Source: CAD feature listing. Evaluate the final solid. Frame: model axes, mm. Face numbers are marked on the shaded views. Give positions to 0.01 mm unless a question says otherwise; leave off trailing zeros. Loops run counter-clockwise (first coordinate to the right, second up) from the corner with the lowest first, then second, coordinate; pieces in that order, holes last.
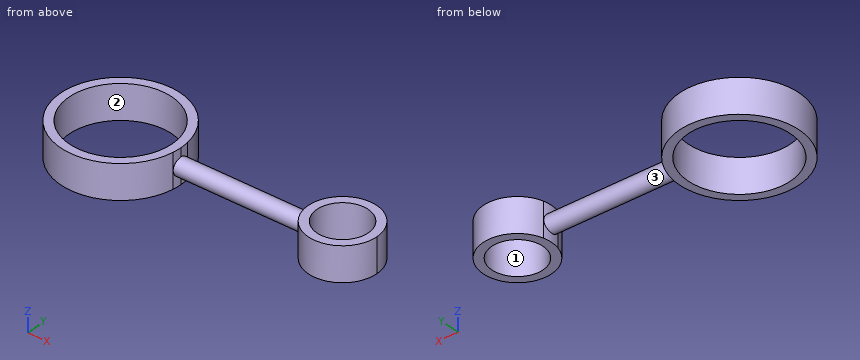
from build123d import *

# Parameters (mm, degrees)
F0_R     = 12.7
F1_DEPTH = 95.25
F2_R     = 76.2
F3_DEPTH = 25.4
F4_R     = 38.1
F5_DEPTH = 25.4


with BuildPart() as f1:
    # F0 (on Right) → F1 (new body, symmetric)
    with BuildSketch(Plane.YZ):
        Circle(F0_R)
    extrude(amount=F1_DEPTH, both=True)

    # F2 (on Top) → F3 (join, symmetric)
    with BuildSketch(Plane.XY):
        with BuildLine():
            ThreePointArc((-94.338181, 0), (-94.566429, 6.366345), (-95.25, 12.7))
            Line((-95.25, 12.7), (-95.25, -12.7))
            ThreePointArc((-95.25, -12.7), (-94.566429, -6.366345), (-94.338181, 0))
        make_face()
        with BuildLine():
            Line((-95.25, -12.7), (-95.25, 12.7))
            ThreePointArc((-95.25, 12.7), (-272.138181, 0), (-95.25, -12.7))
        make_face()
        with Locations((-183.238181, 0)):
            Circle(F2_R, mode=Mode.SUBTRACT)
    extrude(amount=F3_DEPTH, both=True)

    # F4 (on Top) → F5 (join, symmetric)
    with BuildSketch(Plane.XY):
        with BuildLine():
            Line((95.25, -12.7), (95.25, 12.7))
            ThreePointArc((95.25, 12.7), (93.636888, 0), (95.25, -12.7))
        make_face()
        with BuildLine():
            ThreePointArc((195.236888, 0), (150.837907, 50.395109), (95.25, 12.7))
            Line((95.25, 12.7), (95.25, -12.7))
            ThreePointArc((95.25, -12.7), (150.837907, -50.395109), (195.236888, 0))
        make_face()
        with Locations((144.436888, 0)):
            Circle(F4_R, mode=Mode.SUBTRACT)
    extrude(amount=F5_DEPTH, both=True)


solid = f1.part
1) Cut plane A-A (y = 63). Return loops of the section in (x, z), and give its area (3 significant figures).
Checks:
outline: (-245.96, -25.4) - (-226.1, -25.4) - (-226.1, 25.4) - (-245.96, 25.4) - close; (-140.37, -25.4) - (-120.51, -25.4) - (-120.51, 25.4) - (-140.37, 25.4) - close
area: 2,020 mm2
2) Cut plane D-D (z = 6.5). Return loops of the section in (x, y).
Checks:
outline: (-95.25, -12.7) arc R88.9 ccw to (-95.01, -10.91) - (94.82, -10.91) arc R50.8 ccw to (95.25, -12.7) arc R50.8 ccw to (195.24, 0) arc R50.8 ccw to (95.25, 12.7) arc R50.8 ccw to (94.82, 10.91) - (-95.01, 10.91) arc R88.9 ccw to (-95.25, 12.7) arc R88.9 ccw (long way) to start; hole circle Ø152.4 at (-183.24, 0); hole circle Ø76.2 at (144.44, 0)
3) Cut plane B-B (x = -179). Return loops of the section in (y, z), and give its area (3 significant figures).
Checks:
outline: (-88.8, -25.4) - (-76.08, -25.4) - (-76.08, 25.4) - (-88.8, 25.4) - close; (76.08, -25.4) - (88.8, -25.4) - (88.8, 25.4) - (76.08, 25.4) - close
area: 1,290 mm2
4) Contact query for flat-ended pins moving along their axis: P1, Ø12, axis at x = -185, z = -8.5, coming from the +Y side; P2, Ø4, axis at y = -69.5, z = 10, coming from the +X side; P3, Ø12, axis at x = -70.5, z = 14.5, coming from the -Y side. Output: stop coordinate, or through.
Checks:
P1: stops at y = 88.9
P2: stops at x = -125.39
P3: stops at y = -9.44
5) Pull-direction query (Y, two-part tool) for the marked faces 1, 2 and 3; classes: released by +Y, released by -Y, zero draft, split by the parting line, or undercut.
Checks:
face 1: undercut
face 2: undercut
face 3: split by the parting line
6) Cut plane C-C (y = 43). Return loops of the section in (x, z), and give its area (3 significant figures).
Checks:
outline: (-261.05, -25.4) - (-246.15, -25.4) - (-246.15, 25.4) - (-261.05, 25.4) - close; (-120.33, -25.4) - (-105.43, -25.4) - (-105.43, 25.4) - (-120.33, 25.4) - close; (117.39, -25.4) - (171.49, -25.4) - (171.49, 25.4) - (117.39, 25.4) - close
area: 4,260 mm2
7) Ray query, probe 1 along X at (y, z) = (17, -22); probe 2 along Y at (x, z) = (-174.5, 23.5); probe 3 along Y at (x, z) = (123.5, -11.5). Return the intervals inside material, ascending.
Checks:
probe 1: x = -270.5 to -257.52, -108.96 to -95.98, 96.57 to 110.34, 178.53 to 192.31
probe 2: y = -88.47 to -75.7, 75.7 to 88.47
probe 3: y = -46.28 to -31.83, 31.83 to 46.28
